For this review, take the finished solid that the model builds, in its own axes (mm). Face numbers are marked on the shaded views. A direction names the side the tool comes from. Round coordinates to 2 decimals unless told otherwise and drop trailing zeros. Loops run counter-clockwise (first coordinate to the right, second up) from the corner with the lowest first, then second, coordinate; pieces in that order, holes last. Notation, with made-up numbers: (63.25, 53.25) -> (92.25, 53.25) arc R21 ccw to (92.25, 63.25) -> close; hole circle Ø8 at (61, -30). An arc over 180 degrees is marked (long way). Use one line per item in the form item = value. Start each with the question number.
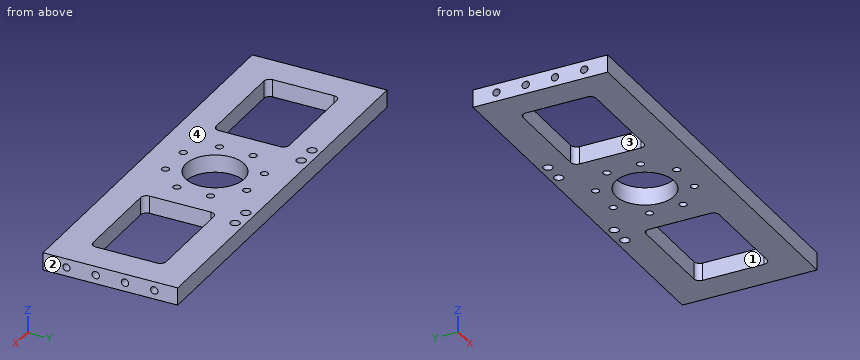
Autodesk Inventor part; units mm, degrees
ref_plane "YZ Plane" through (0, 0, 0) normal (1, 0, 0) x (0, 1, 0)
ref_plane "XZ Plane" through (0, 0, 0) normal (0, 1, 0) x (-1, 0, 0)
ref_plane "XY Plane" through (0, 0, 0) normal (0, 0, 1) x (1, 0, 0)
sketch "스케치1" plane through (0, 0, 0) normal (0, 0, 1) x (1, 0, 0)
  line L0 (0, 0) -> (0, 46)
  line L1 (0, 46) -> (136, 46)
  line L2 (136, 46) -> (136, 0)
  line L3 (136, 0) -> (0, 0)
  dimension "d0" = 46
  dimension "d1" = 136
extrude "돌출1" add sketch "스케치1" along normal blind 6
sketch "스케치2" plane through (0, 0, 6) normal (0, 0, 1) x (1, 0, 0)
  line L0 (0, 46) -> (0, 0)
  line L1 (0, 23) -> (136, 23) construction
  line L2 (136, 0) -> (136, 46)
  line L3 (136, 46) -> (0, 46)
  line L4 (68, 46) -> (68, 0) construction
  line L5 (0, 0) -> (136, 0)
  circle A0 centre (68, 23) radius 14
  line L6 (68, 23) -> (62.2597, 36.8582)
  line L7 (68.3516, 23) -> (83.3516, 23) construction
  circle A1 centre (62.2597, 36.8582) radius 1.25
  circle A2 centre (54.1418, 28.7403) radius 1.25
  circle A3 centre (54.1418, 17.2597) radius 1.25
  circle A4 centre (62.2597, 9.1418) radius 1.25
  circle A5 centre (73.7403, 9.1418) radius 1.25
  circle A6 centre (81.8582, 17.2597) radius 1.25
  circle A7 centre (81.8582, 28.7403) radius 1.25
  circle A8 centre (73.7403, 36.8582) radius 1.25
  circle A9 centre (68, 23) radius 0.245
  dimension "d30" = 28
  dimension "d31" = 15
  dimension "d32" = 112.5
  dimension "d33" = 2.5
  dimension "d34" = 360
extrude "돌출2" cut sketch "스케치2" against normal blind 6 contours A7 A0 | A0 A7 | A6 A0 | A0 A6 | A8 A0 | A0 A8 | A5 A0 | A0 A5 | A1 L6 A0 | A0 A1 | A4 A0 | A0 A4 | L6 A1 A0 | A3 A0 | A0 A3 | A2 A0 | A0 A2
sketch "스케치3" plane through (0, 0, 6) normal (0, 0, 1) x (1, 0, 0)
  line L0 (0, 46) -> (0, 0)
  line L1 (0, 23) -> (136, 23) construction
  line L2 (136, 0) -> (136, 46)
  line L3 (136, 46) -> (0, 46)
  line L4 (68, 46) -> (68, 0) construction
  line L5 (0, 0) -> (136, 0)
  circle A0 centre (68, 23) radius 10
  dimension "d13" = 20
extrude "돌출3" cut sketch "스케치3" against normal blind 6 contours A0
sketch "스케치4" plane through (136, 0, 0) normal (1, 0, 0) x (0, 0, -1)
  line L0 (0, 0) -> (-6, 0)
  line L1 (-3, 0) -> (-3, 46) construction
  line L2 (0, 46) -> (-6, 46)
  circle A0 centre (-3, 38) radius 1.25
  circle A1 centre (-3, 28) radius 1.25
  circle A2 centre (-3, 18) radius 1.25
  circle A3 centre (-3, 8) radius 1.25
  dimension "d16" = 2.5
  dimension "d17" = 2.5
  dimension "d18" = 2.5
  dimension "d19" = 2.5
  dimension "d20" = 10
  dimension "d21" = 10
  dimension "d22" = 10
  dimension "d23" = 8
extrude "돌출4" cut sketch "스케치4" against normal blind 6
sketch "스케치5" plane through (0, 0, 0) normal (-1, 0, 0) x (0, 0, 1)
  line L0 (0, 46) -> (6, 46)
  line L1 (0, 0) -> (6, 0)
  circle A0 centre (3, 38) radius 1.25
  circle A1 centre (3, 28) radius 1.25
  circle A2 centre (3, 18) radius 1.25
  circle A3 centre (3, 8) radius 1.25
extrude "돌출5" cut sketch "스케치5" against normal blind 6
sketch "스케치6" plane through (0, 0, 6) normal (0, 0, 1) x (1, 0, 0)
  circle A0 centre (68, 23) radius 10
  circle A1 centre (81.8582, 17.2597) radius 1.25
  circle A2 centre (54.1418, 28.7403) radius 1.25
  circle A3 centre (54.1418, 17.2597) radius 1.25
  circle A4 centre (73.7403, 36.8582) radius 1.25
  circle A5 centre (73.7403, 9.1418) radius 1.25
  circle A6 centre (62.2597, 36.8582) radius 1.25
  circle A7 centre (62.2597, 9.1418) radius 1.25
  circle A8 centre (81.8582, 28.7403) radius 1.25
  line L0 (136, 46) -> (0, 46)
  line L1 (0, 46) -> (0, 0)
  line L2 (0, 0) -> (136, 0)
  line L3 (136, 0) -> (136, 46)
  line L4 (12.5, 35.5) -> (43.5, 35.5)
  line L5 (45.5, 33.5) -> (45.5, 12.5)
  line L6 (43.5, 10.5) -> (12.5, 10.5)
  line L7 (10.5, 12.5) -> (10.5, 33.5)
  line L8 (136, 46) -> (0, 46)
  line L9 (68, 46) -> (68, 0) construction
  line L10 (0, 0) -> (136, 0)
  line L11 (123.5, 35.5) -> (92.5, 35.5)
  line L12 (90.5, 33.5) -> (90.5, 12.5)
  line L13 (92.5, 10.5) -> (123.5, 10.5)
  line L14 (125.5, 12.5) -> (125.5, 33.5)
  arc A9 (45.5, 33.5) -> (43.5, 35.5) centre (43.5, 33.5) ccw
  arc A10 (43.5, 10.5) -> (45.5, 12.5) centre (43.5, 12.5) ccw
  arc A11 (10.5, 12.5) -> (12.5, 10.5) centre (12.5, 12.5) ccw
  arc A12 (92.5, 35.5) -> (90.5, 33.5) centre (92.5, 33.5) ccw
  arc A13 (125.5, 33.5) -> (123.5, 35.5) centre (123.5, 33.5) ccw
  arc A14 (123.5, 10.5) -> (125.5, 12.5) centre (123.5, 12.5) ccw
  arc A15 (90.5, 12.5) -> (92.5, 10.5) centre (92.5, 12.5) ccw
  arc A16 (12.5, 35.5) -> (10.5, 33.5) centre (12.5, 33.5) ccw
  point P0 (10.5, 35.5)
  point P1 (45.5, 10.5)
  point P2 (45.5, 35.5)
  point P3 (10.5, 10.5)
  point P4 (125.5, 35.5)
  point P5 (90.5, 10.5)
  point P6 (90.5, 35.5)
  point P7 (125.5, 10.5)
  dimension "d35" = 35
  dimension "d36" = 25
  dimension "d37" = 10.5
  dimension "d38" = 10.5
  dimension "d41" = 2
  dimension "d42" = 2
extrude "돌출6" cut sketch "스케치6" against normal blind 6 contours L4 A9 L5 A10 L6 A11 L7 A16 | A13 L14 A14 L13 A15 L12 A12 L11
sketch "스케치11" plane through (0, 0, 6) normal (0, 0, 1) x (1, 0, 0)
  line L0 (136, 46) -> (0, 46)
  line L1 (68, 46) -> (68, 43)
  line L2 (136, 43) -> (0, 43) construction
  circle A0 centre (50, 43) radius 1.6
  circle A1 centre (86, 43) radius 1.6
  circle A2 centre (43, 43) radius 1.6
  circle A3 centre (93, 43) radius 1.6
  point P0 (0, 0)
  dimension "d67" = 3
  dimension "d69" = 3
  dimension "d70" = 3.2
  dimension "d71" = 3.2
  dimension "d72" = 18
  dimension "d73" = 18
  dimension "d74" = 3.2
  dimension "d75" = 3.2
  dimension "d76" = 7
  dimension "d77" = 7
extrude "돌출8" cut sketch "스케치11" against normal blind 10
properties part number "조인트3힌지윗판_6T" material "알루미늄 6061"
Item 1: Take a section at A-A on y = 43. Give the boundary of the cut face in (x, z).
Item 2: Draft analysis for pull direction Y (two halves, no side actions). For the marked faces 1 and 2, state which applies: +Y half, -Y half, draft (parallel to the pull), parting line (faces both ways), or undercut.
Item 3: For P1, Ø3, axis at x = 50, y = 43, coming from the -Z side; P2, Ø2, axis at y = 18, z = 3, coming from the -X side; P3, Ø0.8, axis at y = 28, z = 3, coming from the +X side, all flat-tipped, find the tip position at first contact; note any pin that passes through.
Item 4: Wall thickness on line 1 (Y direction, x = 131.25, z = 3); line 2 (Y direction, x = 119.5, z = 2.25); line 3 (Y direction, x = 68, z = 3.7): over which ranges is each line inside the solid? List them lowest first.
Item 5: Take a section at B-B on x = 86. Give the boundary of the cut face in (y, z), plus the area to 3 significant figures.
Item 6: Take a section at C-C on x = 68. Give the boundary of the cut face in (y, z), plus the area to 3 significant figures.
Item 7: Take a section at D-D on z = 3. Give the number of separate pieces and of enclosed holes in the cut face, plus the area to 3 significant figures.
Item 8: Machinability: for the marked faces 3 and 4, which of the approach directions +Z, -Z, +X, -X, +Y, -Y give a long, thin tool a straight path to every point of the face, cutting with its end or side? Answer none if there is none.
Results:
q1.outline = (0, 0) -> (41.4, 0) -> (41.4, 6) -> (0, 6) -> close; (44.6, 0) -> (48.4, 0) -> (48.4, 6) -> (44.6, 6) -> close; (51.6, 0) -> (84.4, 0) -> (84.4, 6) -> (51.6, 6) -> close; (87.6, 0) -> (91.4, 0) -> (91.4, 6) -> (87.6, 6) -> close; (94.6, 0) -> (136, 0) -> (136, 6) -> (94.6, 6) -> close
q2.face_1 = undercut
q2.face_2 = draft
q3.P1 = through
q3.P2 = 6
q3.P3 = 130
q4.line_1 = 0 to 6.75, 9.25 to 16.75, 19.25 to 26.75, 29.25 to 36.75, 39.25 to 46
q4.line_2 = 0 to 10.5, 35.5 to 46
q4.line_3 = 0 to 13, 33 to 46
q5.outline = (0, 0) -> (41.4, 0) -> (41.4, 6) -> (0, 6) -> close; (44.6, 0) -> (46, 0) -> (46, 6) -> (44.6, 6) -> close
q5.area = 257 mm2
q6.outline = (0, 0) -> (13, 0) -> (13, 6) -> (0, 6) -> close; (33, 0) -> (46, 0) -> (46, 6) -> (33, 6) -> close
q6.area = 156 mm2
q7.separate_pieces = 1
q7.enclosed_holes = 15
q7.area = 4,010 mm2
q8.face_3 = +Z, -Z
q8.face_4 = +Z, +X, -X, +Y, -Y
